CAD build for the part. Positions are in the model's coordinates, mm. Face numbers are marked on the shaded views. A direction names the side the tool comes from. Give positions to 0.01 mm unless a question says otherwise; leave off trailing zeros. Write each loop counter-clockwise with the first axis right and the second up, starting at its lowest first coordinate (ties: lowest second). Pieces come first, ordered by that corner, then holes. Notation, with made-up numbers: (31, 56) - (54, 56) arc R18 ccw to (54, 60) - close; hole circle Ø9 at (72, -13). An arc over 180 degrees is marked (long way). Answer as a JSON object with one key per item and string values.
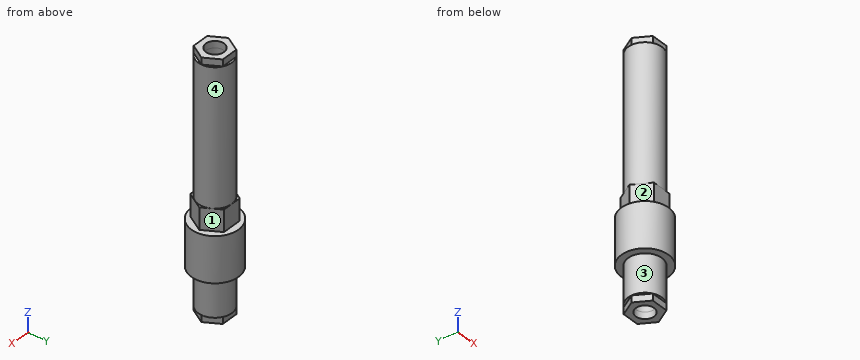
from build123d import *

# Parameters (mm, degrees)
F0_R          = 3.96875
F0_R_2        = 2.15265
F1_DEPTH      = 56.515
F3_R          = 2.15265
F4_DEPTH      = 1.5875
F4_DEPTH_BACK = 58.1025
F6_R          = 5.55625
F6_R_2        = 2.15265
F7_DEPTH      = 10.66165
F8_R          = 2.15265
F9_DEPTH      = 5.08


with BuildPart() as f1:
    # F0 (on Top) → F1 (new body)
    with BuildSketch(Plane.XY):
        Circle(F0_R)
        Circle(F0_R_2, mode=Mode.SUBTRACT)
    extrude(amount=F1_DEPTH)

    # F3 (on face) → F4 (join, two sides)
    with BuildSketch(Plane(origin=(0, 0, 0), x_dir=(1, 0, 0), z_dir=(0, 0, -1))) as f4_sk:
        Polygon((-1.984375, -3.4370383213), (1.984375, -3.4370383213), (3.96875, 0), (1.984375, 3.4370383213), (-1.984375, 3.4370383213), (-3.96875, 0), align=None)
        Circle(F3_R, mode=Mode.SUBTRACT)
    extrude(amount=F4_DEPTH)
    extrude(f4_sk.sketch, amount=-F4_DEPTH_BACK)

    # F6 (on offset) → F7 (join)
    with BuildSketch(Plane(origin=(0, 0, 8.89), x_dir=(1, 0, 0), z_dir=(0, 0, -1))):
        Circle(F6_R)
        Circle(F6_R_2, mode=Mode.SUBTRACT)
    extrude(amount=-F7_DEPTH)

    # F8 (on face) → F9 (join)
    with BuildSketch(Plane.XY.offset(19.55165)):
        Polygon((-2.2913588808, -3.96875), (2.2913588808, -3.96875), (4.5827177617, 0), (2.2913588808, 3.96875), (-2.2913588808, 3.96875), (-4.5827177617, 0), align=None)
        Circle(F8_R, mode=Mode.SUBTRACT)
    extrude(amount=F9_DEPTH)


solid = f1.part
(1) Saw through at B-B, the plane z = 36.5. Give the cut face in (x, y), and give its area (3 significant figures).
Answer key:
{"outline": "circle Ø7.94 at (0, 0); hole circle Ø4.31 at (0, 0)", "area": "34.9 mm²"}
(2) Probe L1, parallel to Y at x = 0, z = 12.25; L2, parallel to Y at x = 0, z = 44.5; L3, parallel to X at y = 0, z = 22.15. List the from-to ranges inside material, lowest first. Write a range as [from, to].
Answer key:
{"L1": "y = [-5.56, -2.15], [2.15, 5.56]", "L2": "y = [-3.97, -2.15], [2.15, 3.97]", "L3": "x = [-4.58, -2.15], [2.15, 4.58]"}
(3) Saw through at A-A, the plane z = 9.5. Give the cut face in (x, y).
Answer key:
{"outline": "circle Ø11.11 at (0, 0); hole circle Ø4.31 at (0, 0)"}
(4) Flat gauge pins, fed straight in: P1, Ø0.8, axis at x = 0.5, z = -0.5, coming from the -Y side; P2, Ø4, axis at y = 0.5, z = 24, coming from the +X side; P3, Ø0.5, axis at x = 0, z = 57.5, coming from the +Y side; P4, Ø2.5, axis at x = 0, y = 0, coming from the -Z side. Where does each tip first touch, or does it go through?
Answer key:
{"P1": "stops at y = -3.44", "P2": "stops at x = 4.58", "P3": "stops at y = 3.44", "P4": "passes through"}
(5) 3-axis set-ups, long thin cutter, end or side, ignore diameter. For the marked faces 1, 2, 3 and 4: which of +Z, -Z, +X, -X, +Y, -Y reach the whole face in a straight line?
Answer key:
{"face 1": "+Z, +X, +Y", "face 2": "+Z, -X, -Y", "face 3": "-Z", "face 4": "+Z"}
